```python
from build123d import *

# Parameters (mm, degrees)
SKETCH1_W           = 5.08
SKETCH1_H           = 25.4
BOSS_EXTRUDE1_DEPTH = 127
SKETCH9_W           = 5.461
SKETCH9_H           = 8.965485494
SKETCH9_W_2         = 5.334
SKETCH9_W_3         = 5.207
SKETCH9_W_4         = 5.08
SKETCH9_W_5         = 4.953
SKETCH9_W_6         = 4.826
CUT_EXTRUDE1_DEPTH  = 12.7


with BuildPart() as part:
    # Sketch1 → Boss-Extrude1 (new body)
    with BuildSketch(Plane.XY):
        with Locations((2.54, 12.7)):
            Rectangle(SKETCH1_W, SKETCH1_H)
    extrude(amount=BOSS_EXTRUDE1_DEPTH)

    # Sketch9 → Cut-Extrude1 (cut)
    with BuildSketch(Plane(origin=(5.08, 0, 0), x_dir=(0, 0, -1), z_dir=(1, 0, 0))):
        with Locations((-15.4305, 20.917257253)):
            Rectangle(SKETCH9_W, SKETCH9_H)
        with Locations((-27.178, 20.917257253)):
            Rectangle(SKETCH9_W_2, SKETCH9_H)
        with Locations((-38.7985, 20.917257253)):
            Rectangle(SKETCH9_W_3, SKETCH9_H)
        with Locations((-56.7055, 20.917257253)):
            Rectangle(SKETCH9_W_3, SKETCH9_H)
        with Locations((-68.199, 20.917257253)):
            Rectangle(SKETCH9_W_4, SKETCH9_H)
        with Locations((-79.5655, 20.917257253)):
            Rectangle(SKETCH9_W_5, SKETCH9_H)
        with Locations((-97.155, 20.917257253)):
            Rectangle(SKETCH9_W_6, SKETCH9_H)
    extrude(amount=-CUT_EXTRUDE1_DEPTH, mode=Mode.SUBTRACT)


solid = part.part
```
Source: CAD feature listing. Evaluate the final solid. Frame: model axes, mm. A direction names the side the tool comes from. Give positions to 0.01 mm unless a question says otherwise; leave off trailing zeros. Loops run counter-clockwise (first coordinate to the right, second up) from the corner with the lowest first, then second, coordinate; pieces in that order, holes last. Notation, with made-up numbers: (16.25, 62) -> (43.25, 62) arc R17 cw to (43.25, 66) -> close; hole circle Ø2 at (53.5, -39). An arc over 180 degrees is marked (long way). Put each result on its own line as item: value. Start each with the question number.
1) Contact query for a flat-ended pin moving along its axis: P1, Ø1.4, axis at x = 2, z = 96.5, coming from the +Y side. Output: stop coordinate, or through.
2) Cut plane A-A (y = 21). State how many separate pieces and enclosed holes the cut face has, then the cut area to 3 significant figures.
3) Cut plane C-C (z = 17). Return loops of the section in (x, y).
4) Material intervals for probe 1 along Y at (x, z) = (3.3, 80), sorted ascending.
5) Draft query along Z for faces 3 (the face through (3, 21, 29.845)), 4 (the face through (3, 0, 63)), 5 (the face through (3, 13, 127)). Return one class per face: released by +Z, released by -Z, zero draft, split by the parting line, or undercut.
6) Reachability of faces 1 (the face through (3, 21, 12.7)), 2 (the face through (0, 13, 63)) from +Z, -Z, +X, -X, +Y, -Y: full face, straight path, thin tool, end or side. Return the list, or none.
Results are:
1. P1: stops at y = 16.43
2. separate pieces: 8
2. enclosed holes: 0
2. area: 462 mm2
3. outline: (0, 0) -> (5.08, 0) -> (5.08, 16.43) -> (0, 16.43) -> close
4. probe 1: y = 0 to 16.43
5. face 3: undercut
5. face 4: zero draft
5. face 5: released by +Z
6. face 1: +X, -X, +Y
6. face 2: +Z, -Z, -X, +Y, -Y
